For this review, take the finished solid that the model builds, in its own axes (mm). Face numbers are marked on the shaded views. A direction names the side the tool comes from. Round coordinates to 2 decimals unless told otherwise and drop trailing zeros. Write each loop counter-clockwise with the first axis right and the second up, starting at its lowest first coordinate (ties: lowest second). Pieces come first, ordered by that corner, then holes.
from build123d import *

# Parameters (mm, degrees)
SKETCH1_W           = 57.552398856
SKETCH1_H           = 35.043016192
BOSS_EXTRUDE1_DEPTH = 16
SKETCH2_R           = 8.540880827
BOSS_EXTRUDE2_DEPTH = 16
SKETCH3_R           = 3.847038177
CUT_EXTRUDE1_DEPTH  = 39


with BuildPart() as part:
    # Sketch1 → Boss-Extrude1 (new body)
    with BuildSketch(Plane.XY):
        Rectangle(SKETCH1_W, SKETCH1_H)
    extrude(amount=BOSS_EXTRUDE1_DEPTH)

    # Sketch2 → Boss-Extrude2 (add)
    with BuildSketch(Plane.XY.offset(16)):
        Circle(SKETCH2_R)
    extrude(amount=BOSS_EXTRUDE2_DEPTH)

    # Sketch3 → Cut-Extrude1 (cut)
    with BuildSketch(Plane.XY.offset(32)):
        Circle(SKETCH3_R)
    extrude(amount=-CUT_EXTRUDE1_DEPTH, mode=Mode.SUBTRACT)


solid = part.part
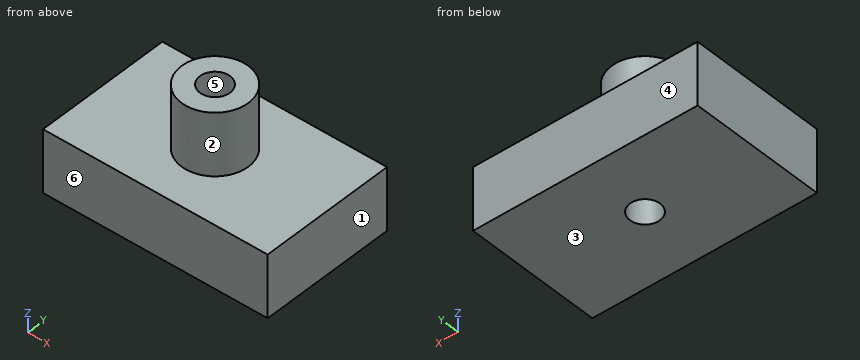
(1) For the marked faces 1 and 2, list the 3-axis set-ups (+Z, -Z, +X, -X, +Y, -Y) from which the entire face can be reached by the end or side of a thin tool; tool diameter is ignored.
Geometry check:
face 1: +Z, -Z, +X, +Y, -Y
face 2: +Z
(2) For line 1 along Z through (x, y) = (-24.5, 15); line 2 along Y through (x, z) = (0, 7); line 3 along Y through (x, z) = (-1.5, 19.5), list the stretches that pass through material, from the lowest coordinate up.
Geometry check:
line 1: z = 0 to 16
line 2: y = -17.52 to -3.85, 3.85 to 17.52
line 3: y = -8.41 to -3.54, 3.54 to 8.41
(3) Mouldability with a two-part tool opening along Y and no side actions: class the marked faces 3, 4, 5 and 6 as pulls with the +Y half, pulls with the -Y half, needs draft (parallel to the pull), parting line crosses it, or undercut.
Geometry check:
face 3: needs draft
face 4: pulls with the +Y half
face 5: undercut
face 6: pulls with the -Y half
(4) We need section A-A, the plane x = 0. Give the boundary of the cut face in (y, z), and give its area (3 significant figures).
Geometry check:
outline: (-17.52, 0) - (-3.85, 0) - (-3.85, 32) - (-8.54, 32) - (-8.54, 16) - (-17.52, 16) - close; (3.85, 0) - (17.52, 0) - (17.52, 16) - (8.54, 16) - (8.54, 32) - (3.85, 32) - close
area: 588 mm2
(5) For pin 1 Ø8 at (y, z) = (-10, 25) entering from -X, flat-tipped, find the tip position at first contact; note if it passes through.
Geometry check:
pin 1: stops at x = -6.08
(6) We need section C-C, the plane z = 3. Give the boundary of the cut face in (x, y), and give its area (3 significant figures).
Geometry check:
outline: (-28.78, -17.52) - (28.78, -17.52) - (28.78, 17.52) - (-28.78, 17.52) - close; hole circle Ø7.69 at (0, 0)
area: 1,970 mm2
(7) We need section D-D, the plane y = -9.5. Give the boundary of the cut face in (x, z), and give its area (3 significant figures).
Geometry check:
outline: (-28.78, 0) - (28.78, 0) - (28.78, 16) - (-28.78, 16) - close
area: 921 mm2
(8) We need section B-B, the plane y = 0. Give the boundary of the cut face in (x, z), and give its area (3 significant figures).
Geometry check:
outline: (-28.78, 0) - (-3.85, 0) - (-3.85, 32) - (-8.54, 32) - (-8.54, 16) - (-28.78, 16) - close; (3.85, 0) - (28.78, 0) - (28.78, 16) - (8.54, 16) - (8.54, 32) - (3.85, 32) - close
area: 948 mm2
